from build123d import *

# Parameters (mm, degrees)
SKETCH1_R           = 2.0701
SKETCH1_R_2         = 14.2875
BOSS_EXTRUDE1_DEPTH = 2.286


with BuildPart() as part:
    # Sketch1 → Boss-Extrude1 (new body)
    with BuildSketch(Plane(origin=(0, 0, 0), x_dir=(-1, 0, 0), z_dir=(0, 0, -1))):
        Polygon((-29.591, 41.275), (-31.75, 39.116), (-31.75, 15.875), (-13.235753401, -19.110856459), (-11.70910986, -20.6375), (11.70910986, -20.6375), (13.235753401, -19.110856459), (31.75, 15.875), (31.75, 39.116), (29.591, 41.275), align=None)
        with Locations((-15.76028553, 9.525)):
            Circle(SKETCH1_R, mode=Mode.SUBTRACT)
        with Locations((9.525, -15.76028553)):
            Circle(SKETCH1_R, mode=Mode.SUBTRACT)
        with Locations((-12.7, 28.575)):
            Circle(SKETCH1_R, mode=Mode.SUBTRACT)
        with Locations((12.7, 28.575)):
            Circle(SKETCH1_R, mode=Mode.SUBTRACT)
        with Locations((25.4, 28.575)):
            Circle(SKETCH1_R, mode=Mode.SUBTRACT)
        Circle(SKETCH1_R_2, mode=Mode.SUBTRACT)
        with Locations((-25.4, 28.575)):
            Circle(SKETCH1_R, mode=Mode.SUBTRACT)
        with Locations((0, 28.575)):
            Circle(SKETCH1_R, mode=Mode.SUBTRACT)
        with Locations((15.76028553, 9.525)):
            Circle(SKETCH1_R, mode=Mode.SUBTRACT)
        with Locations((-9.525, -15.76028553)):
            Circle(SKETCH1_R, mode=Mode.SUBTRACT)
    extrude(amount=-BOSS_EXTRUDE1_DEPTH)


solid = part.part
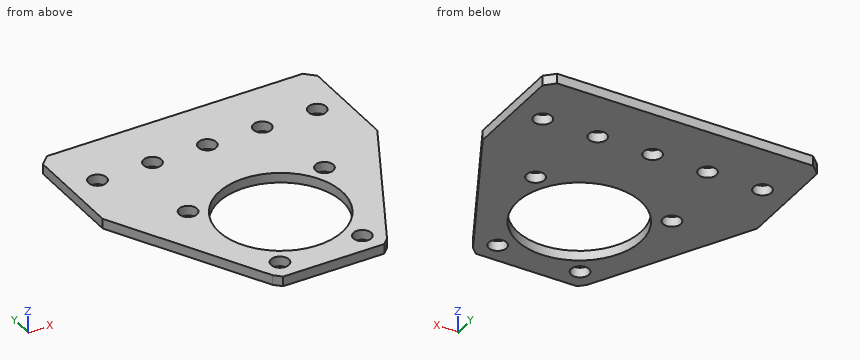
The listing builds one solid part. Answer for the finished solid, in the listing's coordinates (mm). Coordinates: 2 decimals unless noted, no trailing zeros. Write each loop counter-clockwise with the first axis right and the second up, starting at its lowest first coordinate (ties: lowest second). Pieces come first, ordered by that corner, then holes. Notation, with made-up numbers: (68, 75) - (79, 75) arc R26 ccw to (79, 92) - close; hole circle Ø5 at (70, 45.5). An arc over 180 degrees is marked (long way). Return JSON: item names as keys, results as strings.
1. The part is cut by section C-C on x = -25.4. Determine the outline of the cut face in (y, z) (3 decimals).
Final values:
{"outline": "(3.876, 0) - (26.505, 0) - (26.505, 2.286) - (3.876, 2.286) - close; (30.645, 0) - (41.275, 0) - (41.275, 2.286) - (30.645, 2.286) - close"}
2. The part is cut by section D-D on z = 0.45. Count the separate pieces of the cut face and the enclosed holes in it, then the cut area to 3 significant figures.
Final values:
{"separate pieces": "1", "enclosed holes": "10", "area": "2,460 mm^2"}
3. The part is cut by section A-A on x = 0. Determine the outline of the cut face in (y, z) (1 decimal).
Final values:
{"outline": "(-20.6, 0) - (-14.3, 0) - (-14.3, 2.3) - (-20.6, 2.3) - close; (14.3, 0) - (26.5, 0) - (26.5, 2.3) - (14.3, 2.3) - close; (30.6, 0) - (41.3, 0) - (41.3, 2.3) - (30.6, 2.3) - close"}
4. Consider line 1 along Y through (x, z) = (0, 2) (1 decimal); line 2 along X through (y, z) = (10, 2.1); line 3 along Y through (x, z) = (12.7, 1.7) (3 decimals). Determine where each line is inside the solid, lowest interval first.
Final values:
{"line 1": "-20.6 to -14.3, 14.3 to 26.5, 30.6 to 41.3", "line 2": "-28.64 to -17.78, -13.75 to -10.2, 10.2 to 13.75, 17.78 to 28.64", "line 3": "-19.647 to -6.545, 6.545 to 26.505, 30.645 to 41.275"}
5. The part is cut by section B-B on y = -6.5. Determine the outline of the cut face in (x, z), then the cut area to 3 significant figures.
Final values:
{"outline": "(-19.91, 0) - (-12.72, 0) - (-12.72, 2.29) - (-19.91, 2.29) - close; (12.72, 0) - (19.91, 0) - (19.91, 2.29) - (12.72, 2.29) - close", "area": "32.9 mm^2"}
